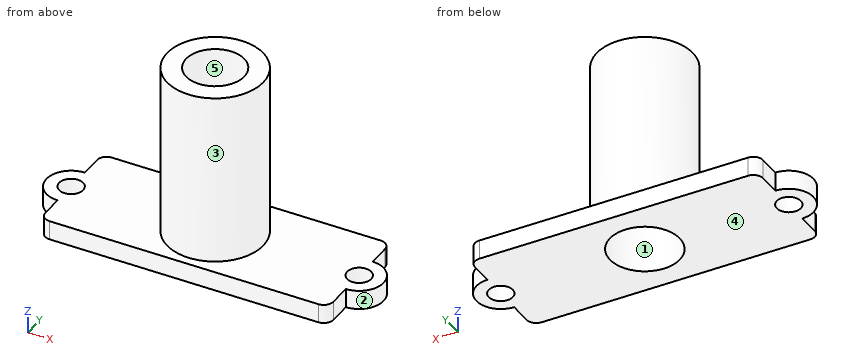
from build123d import *

# Parameters (mm, degrees)
F0_R     = 5
F0_R_2   = 3.6304219053
F0_R_3   = 3.0262783812
F1_DEPTH = 2
F2_DEPTH = 20
F3_D     = 2.5
F3_DEPTH = 10
F3_TIP   = 0.7510757738
F4_DEPTH = 5


with BuildPart() as f1:
    # F0 (on Top) → F1 (new body)
    with BuildSketch(Plane.XY):
        with BuildLine():
            Line((-14, -5.9018372558), (14, -5.9018372558))
            ThreePointArc((14, -5.9018372558), (14.7071067812, -5.608944037), (15, -4.9018372558))
            Line((15, -4.9018372558), (15, -2.5376267174))
            ThreePointArc((15, -2.5376267174), (17.5376267174, 0), (15, 2.5376267174))
            Line((15, 2.5376267174), (15, 4.9018372558))
            ThreePointArc((15, 4.9018372558), (14.7071067812, 5.608944037), (14, 5.9018372558))
            Line((14, 5.9018372558), (-14, 5.9018372558))
            ThreePointArc((-14, 5.9018372558), (-14.7071067812, 5.608944037), (-15, 4.9018372558))
            Line((-15, 4.9018372558), (-15, 2.5700507666))
            ThreePointArc((-15, 2.5700507666), (-17.5700507666, 0), (-15, -2.5700507666))
            Line((-15, -2.5700507666), (-15, -4.9018372558))
            ThreePointArc((-15, -4.9018372558), (-14.7071067812, -5.608944037), (-14, -5.9018372558))
        make_face()
        Circle(F0_R, mode=Mode.SUBTRACT)
        Circle(F0_R)
        Circle(F0_R_2, mode=Mode.SUBTRACT)
        Circle(F0_R_2)
        Circle(F0_R_3, mode=Mode.SUBTRACT)
    extrude(amount=F1_DEPTH)

    # F0 (on Top) → F2 (join)
    with BuildSketch(Plane.XY):
        Circle(F0_R)
        Circle(F0_R_2, mode=Mode.SUBTRACT)
        Circle(F0_R_2)
        Circle(F0_R_3, mode=Mode.SUBTRACT)
    extrude(amount=F2_DEPTH)

    # F3
    with Locations(Plane(origin=(0, 0, 0), x_dir=(1, 0, 0), z_dir=(0, 0, -1))):
        with Locations((-15, 0), (15, 0)):
            Hole(F3_D / 2, depth=F3_DEPTH)
            with Locations((0, 0, -(F3_DEPTH + F3_TIP / 2))):  # 118° drill point
                Cone(0, F3_D / 2, F3_TIP, mode=Mode.SUBTRACT)

    # F0 (on Top) → F4 (cut)
    with BuildSketch(Plane.XY):
        Circle(F0_R_2)
        Circle(F0_R_3, mode=Mode.SUBTRACT)
    extrude(amount=F4_DEPTH, mode=Mode.SUBTRACT)


solid = f1.part
Work out the finished part from the listing and answer in its coordinate system (mm). Face numbers are marked on the shaded views. A direction names the side the tool comes from. Give positions to 0.01 mm unless a question says otherwise; leave off trailing zeros. Order: outer loops, then holes, each group sorted by start corner. A loop starts at its lowest first (then second) coordinate and runs counter-clockwise, first axis right, second up. Notation, with made-up numbers: M -11.75,83 L 29.25,83 A24 cw 29.25,122 Z; hole C 48,6.25 d4. An arc over 180 degrees is marked long. Return JSON: item names as keys, results as strings.
Q1. Find section C-C, the plane y = -2. Write down the section's boundary in (x, z).
Answer below:
{"outline": "M -16.61,0 L -3.03,0 L -3.03,5 L -2.27,5 L -2.27,20 L -4.58,20 L -4.58,2 L -16.61,2 Z; M 2.27,5 L 3.03,5 L 3.03,0 L 16.56,0 L 16.56,2 L 4.58,2 L 4.58,20 L 2.27,20 Z"}
Q2. Each of these flat-tipped pins is pushed along its axis until it touches: pin 1 (1 mm diameter, centred on x = -4, z = 11, fed in from -Y); pin 2 (3.5 mm diameter, centred on x = 0, y = 0, fed in from -Z) (3 decimals); pin 3 (1.6 mm diameter, centred on y = -3.5, z = 1.5, fed in from -X); pin 4 (1.6 mm diameter, centred on y = 3.5, z = 1.5, fed in from +X). Where does it stop, or does it pass through?
Answer below:
{"pin 1": "stops at y = -3.57", "pin 2": "passes through", "pin 3": "stops at x = -15", "pin 4": "stops at x = 15"}
Q3. Find the intervals of material crossed by line 1 along Z through (x, y) = (6.5, 0); line 2 along Y through (x, z) = (0, 3.7); line 3 along X through (y, z) = (-2.25, 1.25), in increasing order. Write a range as [from, to].
Answer below:
{"line 1": "z = [0, 2]", "line 2": "y = [-5, -3.63], [3.63, 5]", "line 3": "x = [-16.24, -2.85], [2.85, 16.17]"}
Q4. Find section A-A, the plane y = 0. Write down the section's boundary in (x, z).
Answer below:
{"outline": "M -17.57,0 L -16.25,0 L -16.25,2 L -17.57,2 Z; M -13.75,0 L -3.63,0 L -3.63,5 L -3.03,5 L -3.03,20 L -5,20 L -5,2 L -13.75,2 Z; M 3.03,5 L 3.63,5 L 3.63,0 L 13.75,0 L 13.75,2 L 5,2 L 5,20 L 3.03,20 Z; M 16.25,0 L 17.54,0 L 17.54,2 L 16.25,2 Z"}
Q5. The mould has two halves that part along X. Classify the marked faces 3, 4 and 5: pulls with the +X half, pulls with the -X half, needs draft (parallel to the pull), parting line crosses it, or undercut.
Answer below:
{"face 3": "parting line crosses it", "face 4": "needs draft", "face 5": "undercut"}
Q6. Find section D-D, the plane z = 12. Write down the section's boundary in (x, y).
Answer below:
{"outline": "C 0,0 d10; hole C 0,0 d6.05"}
Q7. Which of the six approach directions +Z, -Z, +X, -X, +Y, -Y give full straight-line access (tool end or side, diameter ignored) to the marked faces 1 and 2?
Answer below:
{"face 1": "-Z", "face 2": "+Z, -Z, +X"}
Q8. Find section B-B, the plane x = 0. Write down the section's boundary in (y, z), and give its area (3 significant figures).
Answer below:
{"outline": "M -5.9,0 L -3.63,0 L -3.63,5 L -3.03,5 L -3.03,20 L -5,20 L -5,2 L -5.9,2 Z; M 3.03,5 L 3.63,5 L 3.63,0 L 5.9,0 L 5.9,2 L 5,2 L 5,20 L 3.03,20 Z", "area": "76.5 mm^2"}
